```python
from build123d import *

# Parameters (mm, degrees)
F0_R     = 9.525
F1_DEPTH = 12.7
F2_R     = 15.23999


# Not quite as in the source:
# - a fillet or chamfer is up to 0.001 mm smaller than in the source, because OpenCascade refuses the exact size


with BuildPart() as f1:
    # F0 (on Top) → F1 (new body)
    with BuildSketch(Plane.XY):
        Polygon((-15.24, 0), (0, 0), (0, 30.48), (-81.28, 30.48), (-81.28, 0), align=None)
        with Locations((-66.04, 15.24)):
            Circle(F0_R, mode=Mode.SUBTRACT)
        with Locations((-40.64, 15.24)):
            Circle(F0_R, mode=Mode.SUBTRACT)
        with BuildLine():
            ThreePointArc((-5.715, 15.24), (-8.5048079092, 8.5048079092), (-15.24, 5.715))
            ThreePointArc((-15.24, 5.715), (-21.9751920908, 21.9751920908), (-5.715, 15.24))
        make_face(mode=Mode.SUBTRACT)
    extrude(amount=F1_DEPTH)

    # F2 (radius 15.24 in the source; OpenCascade refuses exactly that, so slightly less here)
    f2_edges = [f1.edges().sort_by_distance(p)[0] for p in [
        (0, 0, 6.35),
        (0, 30.48, 6.35),
    ]]
    fillet(f2_edges, radius=F2_R)


solid = f1.part
```
Check sheet for the modelled part. Datum: model origin and axes. Units: mm. Round coordinates to 2 decimals unless told otherwise and drop trailing zeros. Write each loop counter-clockwise with the first axis right and the second up, starting at its lowest first coordinate (ties: lowest second). Pieces come first, ordered by that corner, then holes. Notation, with made-up numbers: (73, 1.25) -> (99, 1.25) arc R9 cw to (99, 8.25) -> close; hole circle Ø9 at (75.25, 59.25). An arc over 180 degrees is marked (long way). One line per question, with ' | ' between items. Start each with the question number.
1. Scan lines: line 1 along Y through (x, z) = (-66.04, 8.5) (3 decimals); line 2 along X through (y, z) = (21.5, 9); line 3 along X through (y, z) = (13, 11.25). Record each from-to range of solid material in increasing order. Write a range as from..to.
2. Sectioned sample at C-C, the plane y = 17. Record the cut outline in (x, z).
3. Sectioned sample at B-B, the plane z = 6.75. Count the separate pieces of the cut face and the enclosed holes in it, then the cut area to 3 significant figures.
4. Release check for a two-part mould opening along Y. For faces 1 (the face through (-4.35, 4.58, 6.44)), 2 (the face through (-48, 30.48, 6)), 3 (the face through (-31.84, 11.59, 6.26)) record: +Y half, -Y half, draft (parallel to the pull), parting line (faces both ways), or undercut.
5. Sectioned sample at D-D, the plane x = -16.5. Record the cut outline in (y, z).
6. Depth check by flat-ended pin: pin 1 (8 mm diameter, centred on x = -11, y = 4.5, fed in from -Z). Enter the tip coordinate at first touch or a pass-through.
7. Sectioned sample at A-A, the plane x = -66.04. Record the cut outline in (y, z) (3 decimals).
Taken from the geometry:
1) line 1: y = 0..5.715, 24.765..30.48 | line 2: x = -81.28..-73.22, -58.86..-47.82, -33.46..-22.42, -8.06..-1.35 | line 3: x = -81.28..-75.3, -56.78..-49.9, -31.38..-24.5, -5.98..-0.17
2) outline: (-81.28, 0) -> (-75.4, 0) -> (-75.4, 12.7) -> (-81.28, 12.7) -> close; (-56.68, 0) -> (-50, 0) -> (-50, 12.7) -> (-56.68, 12.7) -> close; (-31.28, 0) -> (-24.6, 0) -> (-24.6, 12.7) -> (-31.28, 12.7) -> close; (-5.88, 0) -> (-0.1, 0) -> (-0.1, 12.7) -> (-5.88, 12.7) -> close
3) separate pieces: 1 | enclosed holes: 3 | area: 1,520 mm^2
4) face 1: -Y half | face 2: +Y half | face 3: undercut
5) outline: (0, 0) -> (5.8, 0) -> (5.8, 12.7) -> (0, 12.7) -> close; (24.68, 0) -> (30.48, 0) -> (30.48, 12.7) -> (24.68, 12.7) -> close
6) pin 1: stops at z = 0
7) outline: (0, 0) -> (5.715, 0) -> (5.715, 12.7) -> (0, 12.7) -> close; (24.765, 0) -> (30.48, 0) -> (30.48, 12.7) -> (24.765, 12.7) -> close
